from build123d import *

# Parameters (mm, degrees)
BOSS_EXTRUDE1_DEPTH = 15
SKETCH3_R           = 5
CUT_EXTRUDE1_DEPTH  = 3
CUT_EXTRUDE2_START  = -3
SKETCH4_R           = 5
CUT_EXTRUDE2_DEPTH  = 3
SKETCH5_R           = 3.5
CUT_EXTRUDE3_DEPTH  = 64
CUT_EXTRUDE4_DEPTH  = 15
FILLET2_R           = 3
FILLET3_R           = 3
FILLET5_R           = 3
FILLET6_R           = 3
SKETCH7_R           = 1
CUT_EXTRUDE5_DEPTH  = 4


with BuildPart() as part:
    # Sketch2 → Boss-Extrude1 (new body)
    with BuildSketch(Plane(origin=(0, 0, 0), x_dir=(1, 0, 0), z_dir=(0, 1, 0))):
        Polygon((-6, -40), (6, -40), (6, 0), (19.5, 0), (19.5, 40), (13.5, 40), (13.5, 5), (-13.5, 5), (-13.5, 40), (-19.5, 40), (-19.5, 0), (-6, 0), align=None)
    extrude(amount=BOSS_EXTRUDE1_DEPTH)

    # Sketch3 → Cut-Extrude1 (cut)
    with BuildSketch(Plane(origin=(19.5, 0, 0), x_dir=(0, 0, -1), z_dir=(1, 0, 0))):
        with Locations((28, 7.5)):
            Circle(SKETCH3_R)
    extrude(amount=-CUT_EXTRUDE1_DEPTH, mode=Mode.SUBTRACT)

    # Sketch4 → Cut-Extrude2 (cut)
    with BuildSketch(Plane.ZY.offset(19.5).offset(CUT_EXTRUDE2_START)):
        with Locations(Location((-28, 7.5, 0), (0, 0, 180))):
            Circle(SKETCH4_R)
    extrude(amount=CUT_EXTRUDE2_DEPTH, mode=Mode.SUBTRACT)

    # Sketch5 → Cut-Extrude3 (cut)
    with BuildSketch(Plane(origin=(16.5, 0, 0), x_dir=(0, 0, -1), z_dir=(1, 0, 0))):
        with Locations(Location((28, 7.5, 0), (0, 0, 180))):
            Circle(SKETCH5_R)
    extrude(amount=-CUT_EXTRUDE3_DEPTH, mode=Mode.SUBTRACT)

    # Sketch6 → Cut-Extrude4 (cut)
    with BuildSketch(Plane.ZY.offset(6)):
        Polygon((40, 0), (40, 11), (12, 11), (0, 0), align=None)
    extrude(amount=-CUT_EXTRUDE4_DEPTH, mode=Mode.SUBTRACT)

    # Fillet2
    fillet2_edges = [part.edges().sort_by_distance(p)[0] for p in [
        (-16.5, 0, -40),
        (16.5, 0, -40),
        (16.5, 15, -40),
        (-16.5, 15, -40),
    ]]
    fillet(fillet2_edges, radius=FILLET2_R)

    # Fillet3
    fillet3_edges = [part.edges().sort_by_distance(p)[0] for p in [
        (-19.5, 7.5, 0),
        (-13.5, 7.5, -5),
        (13.5, 7.5, -5),
        (19.5, 7.5, 0),
    ]]
    fillet(fillet3_edges, radius=FILLET3_R)

    # Fillet5
    fillet5_edges = [part.edges().sort_by_distance(p)[0] for p in [
        (6, 7.5, 0),
        (-6, 7.5, 0),
        (0, 11, 12),
    ]]
    fillet(fillet5_edges, radius=FILLET5_R)

    # Fillet6
    fillet6_edges = [part.edges().sort_by_distance(p)[0] for p in [
        (6, 13, 40),
        (-6, 13, 40),
    ]]
    fillet(fillet6_edges, radius=FILLET6_R)

    # Sketch7 → Cut-Extrude5 (cut)
    with BuildSketch(Plane.XZ.offset(-11)):
        with Locations(Location((-3.010508875, 37.365518676, 0), (0, 0, 270))):
            Circle(SKETCH7_R)
        with Locations(Location((-3.010508875, 27.365518676, 0), (0, 0, 270))):
            Circle(SKETCH7_R)
        with Locations(Location((-3.010508875, 17.365518676, 0), (0, 0, 270))):
            Circle(SKETCH7_R)
        with Locations(Location((3.010508875, 17.365518676, 0), (0, 0, 90))):
            Circle(SKETCH7_R)
        with Locations(Location((3.010508875, 27.365518676, 0), (0, 0, 90))):
            Circle(SKETCH7_R)
        with Locations(Location((3.010508875, 37.365518676, 0), (0, 0, 90))):
            Circle(SKETCH7_R)
    extrude(amount=-CUT_EXTRUDE5_DEPTH, mode=Mode.SUBTRACT)


solid = part.part
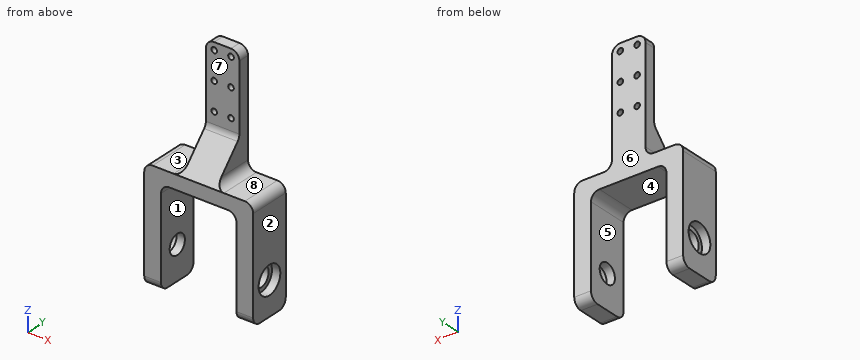
CAD build for the part. Positions are in the model's coordinates, mm. Face numbers are marked on the shaded views. A direction names the side the tool comes from. Give positions to 0.01 mm unless a question says otherwise; leave off trailing zeros. Loops run counter-clockwise (first coordinate to the right, second up) from the corner with the lowest first, then second, coordinate; pieces in that order, holes last. Notation, with made-up numbers: M 66,-31.5 L 97,-31.5 A30 cw 97,1.5 Z; hole C 46.5,23 d6. An arc over 180 degrees is marked long. Answer in a Markdown table with one row per item. Add a question column.
Item 1: Band-saw the part on A-A on z = -28. Give the cut face in (x, y), then the cut area to 3 significant figures.
Item 2: Band-saw the part on B-B on x = 15. Give the cut face in (y, z), then the cut area to 3 significant figures.
Item 3: Tool access for the marked faces 5, 6, 7 and 8: list every direction of +Z, -Z, +X, -X, +Y, -Y with a clear straight run to the whole face (end or side of a thin tool).
Item 4: Band-saw the part on D-D on y = 14.25. Give the cut face in (x, z).
Item 5: Mould opens along X. For the marked faces 1, 2, 3 and 4 say: +X half, -X half, draft (parallel to the pull), parting line (faces both ways), or undercut.
Item 6: Drop flat-ended pins along their axis: P1, Ø6, axis at x = 14, y = 6.5, coming from the +Z side; P2, Ø2.5, axis at x = 3.01, z = 37.37, coming from the -Y side; P3, Ø5, axis at x = 12, y = 10.5, coming from the -Z side; P4, Ø1, axis at x = 0, y = 3.5, coming from the -Z side. Give the stop position or say it passes through.
Item 7: Probe probe 1 along Z at (x, y) = (14.65, 7.5); probe 2 along Y at (x, z) = (-18.25, -28); probe 3 along X at (y, z) = (14.25, 8). List the from-to ranges inside material, lowest first.
Item 8: Band-saw the part on C-C on y = 7.5. Give the number of separate pieces and of enclosed holes in the cut face, then the cut area to 3 significant figures.
Reply:
| question | item | result |
|---|---|---|
| 1 | outline | M -19.5,0 L -13.5,0 L -13.5,4 L -16.5,4 L -16.5,2.5 L -19.5,2.5 Z; M -19.5,12.5 L -16.5,12.5 L -16.5,11 L -13.5,11 L -13.5,15 L -19.5,15 Z; M 13.5,0 L 19.5,0 L 19.5,2.5 L 16.5,2.5 L 16.5,4 L 13.5,4 Z; M 13.5,11 L 16.5,11 L 16.5,12.5 L 19.5,12.5 L 19.5,15 L 13.5,15 Z |
| 1 | area | 78.0 mm^2 |
| 2 | outline | M 0,-37 A3 ccw 3,-40 L 12,-40 A3 ccw 15,-37 L 15,0 L 0,0 Z; hole C 7.5,-28 d7 |
| 2 | area | 558 mm^2 |
| 3 | face 5 | -Z, +Y, -Y |
| 3 | face 6 | +Z, -Z, +X, -X, +Y |
| 3 | face 7 | +Z, +X, -X, -Y |
| 3 | face 8 | +Z, +X, +Y, -Y |
| 4 | outline | M -19.5,-38.98 L -13.5,-38.98 L -13.5,-8 A3 cw -10.5,-5 L 10.5,-5 A3 cw 13.5,-8 L 13.5,-38.98 L 19.5,-38.98 L 19.5,-3 A3 ccw 16.5,0 L 9,0 A3 cw 6,3 L 6,37 A3 ccw 3,40 L -3,40 A3 ccw -6,37 L -6,3 A3 cw -9,0 L -16.5,0 A3 ccw -19.5,-3 Z; hole C -3.01,17.37 d2; hole C -3.01,27.37 d2; hole C -3.01,37.37 d2; hole C 3.01,17.37 d2; hole C 3.01,27.37 d2; hole C 3.01,37.37 d2 |
| 5 | face 1 | undercut |
| 5 | face 2 | +X half |
| 5 | face 3 | draft |
| 5 | face 4 | undercut |
| 6 | P1 | stops at z = 0 |
| 6 | P2 | stops at y = 11 |
| 6 | P3 | stops at z = -40 |
| 6 | P4 | stops at z = -5 |
| 7 | probe 1 | z = -40 to -31.5, -24.5 to 0 |
| 7 | probe 2 | y = 0 to 2.5, 12.5 to 15 |
| 7 | probe 3 | x = -6 to 6 |
| 8 | separate pieces | 3 |
| 8 | enclosed holes | 0 |
| 8 | area | 615 mm^2 |
